Design review of the part built by this model. Coordinates are the model's own, in mm. Give positions to 0.01 mm unless a question says otherwise; leave off trailing zeros. Loops run counter-clockwise (first coordinate to the right, second up) from the corner with the lowest first, then second, coordinate; pieces in that order, holes last. Notation, with made-up numbers: (8, -27.5) -> (17, -27.5) arc R21 ccw to (17, -23.5) -> close; hole circle Ø7 at (-2, -20.75). An arc over 180 degrees is marked (long way). Answer in a Markdown table with one row per item. Add a question column.
(1) Draft analysis for pull direction Y (two halves, no side actions). For faces 1 (the cylindrical face through (2.003, 0.631, 6.533)), 2 (the flat face through (2, -2, 0)), 3 (the cylindrical face through (-0.74, -3.32, 71.7)), 4 (the conical face through (-0.35, 0.11, 13.44)), state which applies: +Y half, -Y half, draft (parallel to the pull), parting line (faces both ways), or undercut.
(2) For pin 1 (3 mm diameter, centred on x = -3.5, z = 46, fed in from -Y); pin 2 (2 mm diameter, centred on x = -4.5, z = 57, fed in from +Y); pin 3 (3 mm diameter, centred on x = 3.5, z = 53, fed in from +Y), all flat-tipped, find the tip position at first contact; note any pin that passes through.
(3) Consider section A-A on z = 10.5. Write out the cut boundary in (x, y).
(4) For line 1 (Y direction, x = 0, z = 4.25); line 2 (Z direction, x = -0.5, y = -3.5); line 3 (Y direction, x = -1.5, z = 14), list the stretches that pass through material, from the lowest coordinate up.
(5) Consider section B-B on z = 64. Write out the cut boundary in (x, y), then the cut area to 3 significant figures.
from build123d import *

# Parameters (mm, degrees)
SKETCH_1_R             = 5.5
EXTRUDE_1_DEPTH        = 68
CHAMFER_1_SIZE         = 0.5
SKETCH_2_R             = 3.4
EXTRUDE_2_DEPTH        = 8
CHAMFER_2_SIZE         = 0.5
HOLE_WIZARD_M5_1_D     = 4.2
HOLE_WIZARD_M5_1_DEPTH = 12.4
HOLE_WIZARD_M5_1_TIP   = 1.2618073
CHAMFER_3_SIZE         = 0.5


with BuildPart() as part:
    # 草图1 → 拉伸1 (new body)
    with BuildSketch(Plane.XY):
        Circle(SKETCH_1_R)
    extrude(amount=EXTRUDE_1_DEPTH)

    # 倒角1
    chamfer_1_edges = [part.edges().sort_by_distance(p)[0] for p in [
        (-5.5, 0, 0),
        (-5.5, 0, 68),
    ]]
    chamfer(chamfer_1_edges, length=CHAMFER_1_SIZE)

    # 草图2 → 拉伸2 (add)
    with BuildSketch(Plane.XY.offset(68)):
        Circle(SKETCH_2_R)
    extrude(amount=EXTRUDE_2_DEPTH)

    # 倒角2
    chamfer_2_edges = [part.edges().sort_by_distance(p)[0] for p in [
        (-3.4, 0, 76),
    ]]
    chamfer(chamfer_2_edges, length=CHAMFER_2_SIZE)

    # M5 螺纹孔1
    with Locations(Plane(origin=(0, 0, 0), x_dir=(-1, 0, 0), z_dir=(0, 0, -1))):
        with Locations((0, 0)):
            Hole(HOLE_WIZARD_M5_1_D / 2, depth=HOLE_WIZARD_M5_1_DEPTH)
            with Locations((0, 0, -(HOLE_WIZARD_M5_1_DEPTH + HOLE_WIZARD_M5_1_TIP / 2))):  # 118° drill point
                Cone(0, HOLE_WIZARD_M5_1_D / 2, HOLE_WIZARD_M5_1_TIP, mode=Mode.SUBTRACT)

    # 倒角3
    chamfer_3_edges = [part.edges().sort_by_distance(p)[0] for p in [
        (-2.1, 0, 0),
    ]]
    chamfer(chamfer_3_edges, length=CHAMFER_3_SIZE)


solid = part.part
Values follow:
| question | item | result |
|---|---|---|
| 1 | face 1 | undercut |
| 1 | face 2 | draft |
| 1 | face 3 | parting line |
| 1 | face 4 | undercut |
| 2 | pin 1 | y = -5.12 |
| 2 | pin 2 | y = 4.24 |
| 2 | pin 3 | y = 5.12 |
| 3 | outline | circle Ø11 at (0, 0); hole circle Ø4.2 at (0, 0) |
| 4 | line 1 | -5.5 to -2.1, 2.1 to 5.5 |
| 4 | line 2 | 0 to 68 |
| 4 | line 3 | -5.29 to 5.29 |
| 5 | outline | circle Ø11 at (0, 0) |
| 5 | area | 95.0 mm2 |
